```python
from build123d import *

# Parameters (mm, degrees)
SKETCH1_W           = 25.4
SKETCH1_H           = 25.4
BOSS_EXTRUDE1_DEPTH = 127
FILLET1_R           = 1.5875
HOLE1_OUTLINE_R     = 2.5527
HOLE1_DEPTH         = 127
SKETCH7_W           = 6.5278
SKETCH7_H           = 2.2352
CUT_EXTRUDE2_DEPTH  = 127
FILLET4_R           = 0.396875
CIRPATTERN2_DEPTH   = 127


# Read off the part's stored shape, not the designer's step: Hole1, CirPattern2
with BuildPart() as part:
    # Sketch1 → Boss-Extrude1 (new body)
    with BuildSketch(Plane.XY):
        Rectangle(SKETCH1_W, SKETCH1_H)
    extrude(amount=BOSS_EXTRUDE1_DEPTH)

    # Fillet1
    fillet1_edges = [part.edges().sort_by_distance(p)[0] for p in [
        (12.7, -12.7, 63.5),
        (-12.7, -12.7, 63.5),
        (-12.7, 12.7, 63.5),
        (12.7, 12.7, 63.5),
    ]]
    fillet(fillet1_edges, radius=FILLET1_R)

    # Hole1 outline → Hole1 (cut)
    with BuildSketch(Plane.XY):
        with Locations((0, -0.048792482)):
            Circle(HOLE1_OUTLINE_R)
    extrude(amount=HOLE1_DEPTH, mode=Mode.SUBTRACT)

    # Sketch7 → Cut-Extrude2 (cut)
    with BuildSketch(Plane.XY.offset(127)):
        with Locations((0, 11.5824)):
            Rectangle(SKETCH7_W, SKETCH7_H)
        Polygon((-3.175, 4.5212), (-7.3025, 10.4648), (7.3025, 10.4648), (3.175, 4.5212), align=None)
    extrude(amount=-CUT_EXTRUDE2_DEPTH, mode=Mode.SUBTRACT)

    # Fillet4
    fillet4_edges = [part.edges().sort_by_distance(p)[0] for p in [
        (-3.2639, 10.4648, 63.5),
        (-3.2639, 12.7, 63.5),
        (3.2639, 12.7, 63.5),
        (3.2639, 10.4648, 63.5),
    ]]
    fillet(fillet4_edges, radius=FILLET4_R)

    # CirPattern2 outline → CirPattern2 (cut)
    with BuildSketch(Plane.XY):
        with BuildLine():
            ThreePointArc((-3.660775, -10.562384964), (-3.380141996, -10.67862696), (-3.2639, -10.959259964))
            Line((-3.2639, -10.959259964), (-3.2639, -12.7))
            Line((-3.2639, -12.7), (3.2639, -12.7))
            Line((3.2639, -12.7), (3.2639, -10.959259964))
            ThreePointArc((3.2639, -10.959259964), (3.380141996, -10.67862696), (3.660775, -10.562384964))
            Line((3.660775, -10.562384964), (7.3025, -10.562384964))
            Line((7.3025, -10.562384964), (3.175, -4.618784964))
            Line((3.175, -4.618784964), (-3.175, -4.618784964))
            Line((-3.175, -4.618784964), (-7.3025, -10.562384964))
            Line((-7.3025, -10.562384964), (-3.660775, -10.562384964))
        make_face()
        with BuildLine():
            Line((-12.7, -3.312692482), (-10.910467482, -3.312692482))
            ThreePointArc((-10.910467482, -3.312692482), (-10.629834478, -3.428934478), (-10.513592482, -3.709567482))
            Line((-10.513592482, -3.709567482), (-10.513592482, -7.351292482))
            Line((-10.513592482, -7.351292482), (-4.569992482, -3.223792482))
            Line((-4.569992482, -3.223792482), (-4.569992482, 3.126207518))
            Line((-4.569992482, 3.126207518), (-10.513592482, 7.253707518))
            Line((-10.513592482, 7.253707518), (-10.513592482, 3.611982518))
            ThreePointArc((-10.513592482, 3.611982518), (-10.629834478, 3.331349514), (-10.910467482, 3.215107518))
            Line((-10.910467482, 3.215107518), (-12.7, 3.215107518))
            Line((-12.7, 3.215107518), (-12.7, -3.312692482))
        make_face()
        with BuildLine():
            ThreePointArc((10.513592482, -3.709567482), (10.629834478, -3.428934478), (10.910467482, -3.312692482))
            Line((10.910467482, -3.312692482), (12.7, -3.312692482))
            Line((12.7, -3.312692482), (12.7, 3.215107518))
            Line((12.7, 3.215107518), (10.910467482, 3.215107518))
            ThreePointArc((10.910467482, 3.215107518), (10.629834478, 3.331349514), (10.513592482, 3.611982518))
            Line((10.513592482, 3.611982518), (10.513592482, 7.253707518))
            Line((10.513592482, 7.253707518), (4.569992482, 3.126207518))
            Line((4.569992482, 3.126207518), (4.569992482, -3.223792482))
            Line((4.569992482, -3.223792482), (10.513592482, -7.351292482))
            Line((10.513592482, -7.351292482), (10.513592482, -3.709567482))
        make_face()
    extrude(amount=CIRPATTERN2_DEPTH, mode=Mode.SUBTRACT)


solid = part.part
```
Model file for the job. Use its own axes, mm. A direction names the side the tool comes from. Coordinates: 2 decimals unless noted, no trailing zeros. Order: outer loops, then holes, each group sorted by start corner. A loop starts at its lowest first (then second) coordinate and runs counter-clockwise, first axis right, second up. Notation, with made-up numbers: (43.25, 29.25) -> (80.25, 29.25) arc R11 cw to (80.25, 38.25) -> close; hole circle Ø7 at (64, 5.25). An arc over 180 degrees is marked (long way). Return JSON: item names as keys, results as strings.
Item 1: 3-axis set-ups, long thin cutter, end or side, ignore diameter. For faces 4 (the face through (4.57, 0, 63)), 5 (the face through (0, 4.521, 64)), 6 (the face through (7.583, 5.219, 62.611)): which of +Z, -Z, +X, -X, +Y, -Y reach the whole face in a straight line?
Model answer:
{"face 4": "+Z, -Z, +X", "face 5": "+Z, -Z, +Y", "face 6": "+Z, -Z"}
Item 2: Pin check, flat tips, straight feed: P1, Ø1.4, axis at y = -11.5, z = 54, coming from the +X side; P2, Ø6, axis at x = 0, z = 94, coming from the -Y side; P3, Ø4, axis at y = -0.5, z = 93.5, coming from the -X side; P4, Ø3, axis at y = -0.5, z = 76, coming from the +X side. Stop position of each tip, or through.
Model answer:
{"P1": "stops at x = 12.7", "P2": "stops at y = -4.62", "P3": "stops at x = -4.57", "P4": "stops at x = 4.57"}
Item 3: Wall check: line 1 along X through (y, z) = (-4.75, 96); line 2 along Y through (x, z) = (0, 53); line 3 along Y through (x, z) = (3.5, 103.5). Give the ranges that are in metal, low to high. Write a range as from..to.
Model answer:
{"line 1": "x = -12.7..-10.51, -6.77..-3.27, 3.27..6.77, 10.51..12.7", "line 2": "y = -4.62..-2.6, 2.5..4.52", "line 3": "y = -12.7..-10.6, -5.09..4.99, 10.5..12.67"}
Item 4: Slice it at B-B (y = 1.25). Write the cut outline in (x, z), then the cut area to 3 significant figures.
Model answer:
{"outline": "(-4.57, 0) -> (-2.2, 0) -> (-2.2, 127) -> (-4.57, 127) -> close; (2.2, 0) -> (4.57, 0) -> (4.57, 127) -> (2.2, 127) -> close", "area": "603 mm²"}
Item 5: Slice it at A-A (x = 0). Write the cut outline in (y, z).
Model answer:
{"outline": "(-4.62, 0) -> (-2.6, 0) -> (-2.6, 127) -> (-4.62, 127) -> close; (2.5, 0) -> (4.52, 0) -> (4.52, 127) -> (2.5, 127) -> close"}
Item 6: Mould opens along Y. For faces 1 (the face through (1.2, -2.3, 62.6)), 2 (the face through (-12.7, -7, 63)), 3 (the face through (0, -4.619, 63)) say: pulls with the +Y half, pulls with the -Y half, needs draft (parallel to the pull), parting line crosses it, or undercut.
Model answer:
{"face 1": "undercut", "face 2": "needs draft", "face 3": "pulls with the -Y half"}
